Design review of the part shown in the three views and the two pictorial views. Dimensions are in mm from the part's minimum x, y and z. A direction names the side the tool comes from. Coordinates: 2 decimals unless noted, no trailing zeros. Loops run counter-clockwise (first coordinate to the right, second up) from the corner with the lowest first, then second, coordinate; pieces in that order, holes last. Notation, with made-up numbers: M -22.5,24 L 11.5,24 A5 ccw 11.5,29 Z; hole C -20,69.5 d3. An arc over 180 degrees is marked long. Answer as a JSON object with one key per item and string values. Group by question number.
Item 1: Wall thickness on L1, parallel to Z at x = 7.9, y = 1.9; L2, parallel to X at y = 1.95, z = 6.5; L3, parallel to X at y = 1.85, z = 4: over which ranges is each line inside the solid? List them lowest first. Write a range as from..to.
Item 2: Mouldability with a two-part tool opening along Z and no side actions: class the marked faces 1, 2 and 3 as +Z half, -Z half, draft (parallel to the pull), parting line (faces both ways), or undercut.
Item 3: Add section B-B (x = 7.9). State the section outline as (y, z) points.
Item 4: Add section A-A (y = 0.75). State the section outline as (x, z) points, then the cut area to 3 significant figures.
Item 5: Tool access review of the marked faces 4, 5 and 6: name each direction out of +Z, -Z, +X, -X, +Y, -Y from which nothing blocks a thin tool from reaching the whole face with its end or side.
Item 6: Add section D-D (y = 2.7). State the section outline as (x, z) points.
Item 7: Add section C-C (z = 6.5). State the section outline as (x, y) points.
Item 8: Insertion check: pin 1 (1.2 mm diameter, centred on x = 7.5, z = 4.5, fed in from -Y); pin 2 (2.5 mm diameter, centred on x = 12.5, z = 4.5, fed in from -Y); pin 3 (1.4 mm diameter, centred on x = 11.9, z = 4, fed in from -Y). Each pin has a flat end and moves straight along its axis. Give the tip position at first contact, or say it passes through.
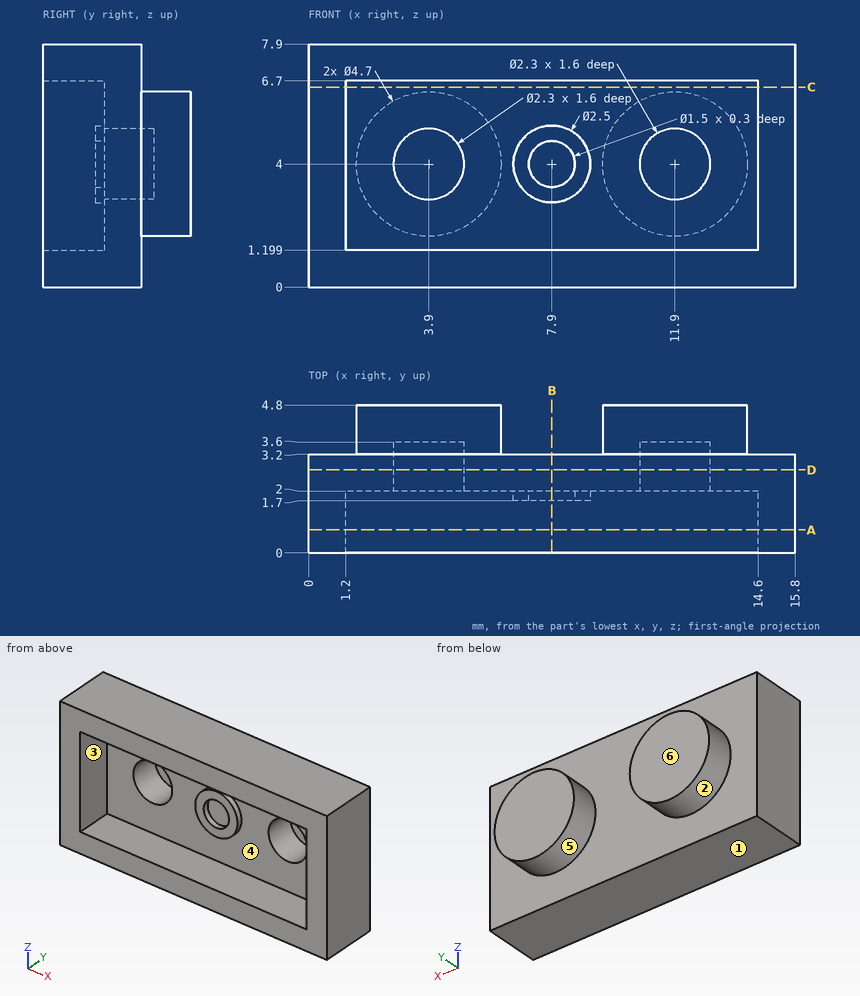
From the geometry:
{
 "1": {"L1": "z = 0..1.2, 2.75..3.25, 4.75..5.25, 6.7..7.9", "L2": "x = 0..1.2, 14.6..15.8", "L3": "x = 0..1.2, 6.65..7.15, 8.65..9.15, 14.6..15.8"},
 "2": {"face 1": "-Z half", "face 2": "parting line", "face 3": "undercut"},
 "3": {"outline": "M 0,0 L 3.2,0 L 3.2,7.9 L 0,7.9 L 0,6.7 L 2,6.7 L 2,5.25 L 1.7,5.25 L 1.7,4.75 L 2,4.75 L 2,3.25 L 1.7,3.25 L 1.7,2.75 L 2,2.75 L 2,1.2 L 0,1.2 Z"},
 "4": {"outline": "M 0,0 L 15.8,0 L 15.8,7.9 L 0,7.9 Z; hole M 1.2,1.2 L 14.6,1.2 L 14.6,6.7 L 1.2,6.7 Z", "area": "51.1 mm²"},
 "5": {"face 4": "-Y", "face 5": "+Y", "face 6": "+Z, -Z, +X, -X, +Y"},
 "6": {"outline": "M 0,0 L 15.8,0 L 15.8,7.9 L 0,7.9 Z; hole C 3.9,4 d2.3; hole C 11.9,4 d2.3"},
 "7": {"outline": "M 0,0 L 1.2,0 L 1.2,2 L 14.6,2 L 14.6,0 L 15.8,0 L 15.8,3.2 L 0,3.2 Z"},
 "8": {"pin 1": "stops at y = 1.7", "pin 2": "stops at y = 2", "pin 3": "stops at y = 3.6"}
}
